```python
from build123d import *

# Parameters (mm, degrees)
SKETCH_1_W          = 30
SKETCH_1_H          = 40
EXTRUDE_1_DEPTH     = 8
SKETCH_2_R          = 4.38634244
SKETCH_2_R_2        = 1.8
EXTRUDE_2_DEPTH     = 40
SKETCH_3_R          = 1.6
CUT_EXTRUDE_1_DEPTH = 9.38634244
SKETCH_4_W          = 22
SKETCH_4_H          = 12
CUT_EXTRUDE_2_DEPTH = 9.38634244


with BuildPart() as part:
    # 草图1 → 凸台-拉伸1 (new body)
    with BuildSketch(Plane(origin=(0, 0, 0), x_dir=(1, 0, 0), z_dir=(0, 1, 0))):
        with Locations((36.36947716, -2.04637122)):
            Rectangle(SKETCH_1_W, SKETCH_1_H)
    extrude(amount=EXTRUDE_1_DEPTH)

    # 草图2 → 凸台-拉伸2 (add)
    with BuildSketch(Plane.XY.offset(22.04637122)):
        with Locations((53.16947716, 4)):
            Circle(SKETCH_2_R)
        with Locations((53.16947716, 4)):
            Circle(SKETCH_2_R_2, mode=Mode.SUBTRACT)
    extrude(amount=-EXTRUDE_2_DEPTH)

    # 草图3 → 切除-拉伸1 (cut, through all)
    with BuildSketch(Plane(origin=(0, 8, 0), x_dir=(1, 0, 0), z_dir=(0, 1, 0))):
        with Locations((26.36947716, 9.95362878)):
            Circle(SKETCH_3_R)
        with Locations((43.36947716, 9.95362878)):
            Circle(SKETCH_3_R)
        with Locations((43.36947716, -14.04637122)):
            Circle(SKETCH_3_R)
        with Locations((26.36947716, -14.04637122)):
            Circle(SKETCH_3_R)
    extrude(amount=-CUT_EXTRUDE_1_DEPTH, mode=Mode.SUBTRACT)

    # 草图4 → 切除-拉伸2 (cut, through all)
    with BuildSketch(Plane(origin=(0, 8, 0), x_dir=(1, 0, 0), z_dir=(0, 1, 0))):
        with Locations((37.36947716, -2.04637122)):
            Rectangle(SKETCH_4_W, SKETCH_4_H)
    extrude(amount=-CUT_EXTRUDE_2_DEPTH, mode=Mode.SUBTRACT)


solid = part.part
```
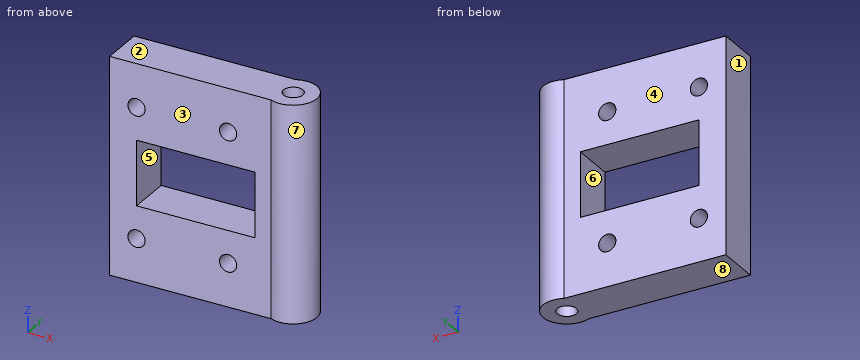
Source: CAD feature listing. Evaluate the final solid. Frame: model axes, mm. Face numbers are marked on the shaded views. A direction names the side the tool comes from. Coordinates: 2 decimals unless noted, no trailing zeros. Write each loop counter-clockwise with the first axis right and the second up, starting at its lowest first coordinate (ties: lowest second). Pieces come first, ordered by that corner, then holes. Notation, with made-up numbers: (2, -22) -> (38, -22) arc R18 ccw to (38, -17) -> close; hole circle Ø6 at (-2.75, -14). An arc over 180 degrees is marked (long way). Return JSON: item names as keys, results as strings. Group by question number.
1) Section query D-D, the plane y = 6.5. Return loops of the section in (x, z).
2) Section query C-C, the plane x = 46.5. Return loops of the section in (y, z).
3) Contact query for flat-ended pins moving along their axis: P1, Ø3.5, axis at x = 43.37, z = 14.05, coming from the +Y side; P2, Ø9, axis at x = 36.5, z = 11.5, coming from the -Y side; P3, Ø2, axis at x = 28.5, z = 4, coming from the -Y side. Output: stop coordinate, or through.
4) Set-up query: the marked faces 1, 2, 3, 4 and 5. Return all of +Z, -Z, +X, -X, +Y, -Y with unobstructed straight access to the full face (end or side cutting, diameter ignored); none if empty.
5) Ray query, line 1 along X through (y, z) = (4, 2); line 2 along Z through (x, y) = (27, 2); line 3 along X through (y, z) = (4, 11.5). Return the intervals inside material, ascending.
6) Section query A-A, the plane z = 3.5. Return loops of the section in (x, y).
7) Mould query, pull axis Z, two halves, no side actions, for the marked faces 6, 7 and 8. Classes: +Z half, -Z half, draft (parallel to the pull), parting line (faces both ways), or undercut.
8) Section query B-B, the plane y = 4. Return loops of the section in (x, z).
From the geometry:
{
 "1": {"outline": "(21.37, -17.95) -> (56.77, -17.95) -> (56.77, 22.05) -> (21.37, 22.05) -> close; hole circle Ø3.2 at (26.37, -9.95); hole circle Ø3.2 at (26.37, 14.05); hole (26.37, -3.95) -> (48.37, -3.95) -> (48.37, 8.05) -> (26.37, 8.05) -> close; hole circle Ø3.2 at (43.37, -9.95); hole circle Ø3.2 at (43.37, 14.05)"},
 "2": {"outline": "(0, -17.95) -> (8, -17.95) -> (8, -3.95) -> (0, -3.95) -> close; (0, 8.05) -> (8, 8.05) -> (8, 22.05) -> (0, 22.05) -> close"},
 "3": {"P1": "y = 8", "P2": "y = 0", "P3": "through"},
 "4": {"face 1": "+Z, -Z, -X, +Y, -Y", "face 2": "+Z, +X, -X, +Y, -Y", "face 3": "+Z, -Z, -X, -Y", "face 4": "+Z, -Z, -X, +Y", "face 5": "+Y, -Y"},
 "5": {"line 1": "21.37 to 26.37, 48.37 to 51.37, 54.97 to 57.56", "line 2": "-17.95 to -11.42, -8.48 to -3.95, 8.05 to 12.58, 15.52 to 22.05", "line 3": "21.37 to 51.37, 54.97 to 57.56"},
 "6": {"outline": "(21.37, 0) -> (26.37, 0) -> (26.37, 8) -> (21.37, 8) -> close; (48.37, 0) -> (51.37, 0) arc R4.39 ccw (long way) to (51.37, 8) -> (48.37, 8) -> close; hole circle Ø3.6 at (53.17, 4)"},
 "7": {"face 6": "undercut", "face 7": "draft", "face 8": "-Z half"},
 "8": {"outline": "(21.37, -17.95) -> (51.37, -17.95) -> (51.37, 22.05) -> (21.37, 22.05) -> close; (54.97, -17.95) -> (57.56, -17.95) -> (57.56, 22.05) -> (54.97, 22.05) -> close; hole circle Ø3.2 at (26.37, -9.95); hole circle Ø3.2 at (26.37, 14.05); hole (26.37, -3.95) -> (48.37, -3.95) -> (48.37, 8.05) -> (26.37, 8.05) -> close; hole circle Ø3.2 at (43.37, -9.95); hole circle Ø3.2 at (43.37, 14.05)"}
}
